Could you check a few things on this drawing? It's one solid part, dimensions in mm from its lowest x, y, z. A direction names the side the tool comes from. Coordinates: 2 decimals unless noted, no trailing zeros. Write each loop counter-clockwise with the first axis right and the second up, starting at its lowest first coordinate (ties: lowest second). Pieces come first, ordered by that corner, then holes. Notation, with made-up numbers: (80, 7.5) - (94, 7.5) arc R17 cw to (94, 19.5) - close; hole circle Ø2 at (-4.75, 16). An arc over 180 degrees is marked (long way). Write item = value, one per line. Start each with the question number.
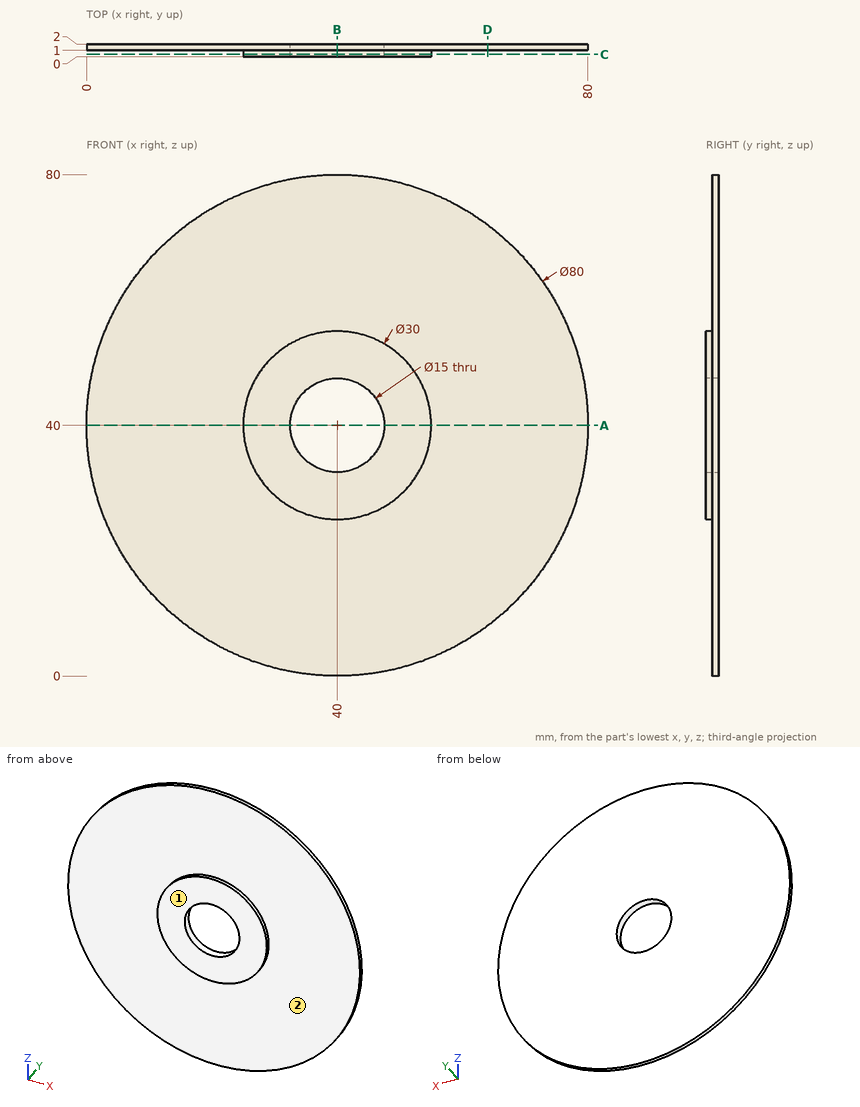
1) Suppose I cut it at B-B on x = 40. Please give me the cut outline in (y, z).
2) Suppose I cut it at D-D on x = 64. Please give me the cut outline in (y, z), plus the area to 3 significant figures.
3) If I drill on probe 1 along X at (y, z) = (1.45, 40); probe 2 along X at (y, z) = (0.9, 40); probe 3 along Z at (x, y) = (45, 0.85), over which ranges is the centre line in solid material (lowest first)? Write a range as [from, to].
4) Suppose I cut it at C-C on y = 0.35. Please give me the cut outline in (x, z), plus the area to 3 significant figures.
5) Suppose I cut it at A-A on z = 40. Please give me the cut outline in (x, y).
6) For P1, Ø3, axis at x = 55, z = 67, coming from the -Y side, with a flat end and sliding along its axis, tell me the tip position at first contact or that it passes through.
7) Which directions (+Z, -Z, +X, -X, +Y, -Y) give clear straight access to the entire face, cutting with the end or side of a thin tool? Please do the marked faces 1 and 2.
Reply:
q1.outline = (0, 25) - (1, 25) - (1, 0) - (2, 0) - (2, 32.5) - (0, 32.5) - close; (0, 47.5) - (2, 47.5) - (2, 80) - (1, 80) - (1, 55) - (0, 55) - close
q2.outline = (1, 8) - (2, 8) - (2, 72) - (1, 72) - close
q2.area = 64.0 mm^2
q3.probe_1 = [0, 32.5], [47.5, 80]
q3.probe_2 = [25, 32.5], [47.5, 55]
q3.probe_3 = [25.86, 34.41], [45.59, 54.14]
q4.outline = circle Ø30 at (40, 40); hole circle Ø15 at (40, 40)
q4.area = 530 mm^2
q5.outline = (0, 1) - (25, 1) - (25, 0) - (32.5, 0) - (32.5, 2) - (0, 2) - close; (47.5, 0) - (55, 0) - (55, 1) - (80, 1) - (80, 2) - (47.5, 2) - close
q6.P1 = 1
q7.face_1 = +Z, -Z, +X, -X, -Y
q7.face_2 = -Y
